from build123d import *

# Parameters (mm, degrees)
BOX008_W               = 22.5
BOX008_H               = 3
BOX008_DEPTH           = 95
BOX009_W               = 6
BOX009_H               = 25
BOX009_DEPTH           = 95
CYLINDER012_R          = 12.5
CYLINDER012_DEPTH      = 13
CYLINDER012_ROLL_ANGLE = 90


with BuildPart() as cube008:
    # Box008 → Box008 (new body)
    with BuildSketch(Plane(origin=(-7.5, 19, 0), x_dir=(1, 0, 0), z_dir=(0, 0, 1))):
        with Locations((11.25, 1.5)):
            Rectangle(BOX008_W, BOX008_H)
    extrude(amount=BOX008_DEPTH)


with BuildPart() as cube009:
    # Box009 → Box009 (new body)
    with BuildSketch(Plane(origin=(0.75, 0, 0), x_dir=(1, 0, 0), z_dir=(0, 0, 1))):
        with Locations((3, 12.5)):
            Rectangle(BOX009_W, BOX009_H)
    extrude(amount=BOX009_DEPTH)


with BuildPart() as obj1:
    # Cylinder012 → Cylinder012 (new body)
    with BuildSketch(Plane.XY):
        Circle(CYLINDER012_R)
    extrude(amount=CYLINDER012_DEPTH)


with BuildPart() as obj1_1:
    # Cylinder012 roll: moved
    add(obj1.part.rotate(Axis((0, 0, 0), (1, 0, 0)), CYLINDER012_ROLL_ANGLE))


with BuildPart() as obj1_2:
    # Cylinder012 placement: moved
    add(obj1_1.part.moved(Location((3.75, 22, 96.2))))

    # Fusion017: union Cube008, Cube009
    add(cube008.part)
    add(cube009.part)


solid = obj1_2.part
Verification items for the finished model (mm, model axes). A direction names the side the tool comes from. Coordinates: 2 decimals unless noted, no trailing zeros. Loops run counter-clockwise (first coordinate to the right, second up) from the corner with the lowest first, then second, coordinate; pieces in that order, holes last. Notation, with made-up numbers: M 43,13 L 90,13 A5 cw 90,22 Z; hole C -30.5,56 d11. An arc over 180 degrees is marked long. One line per item, written item: value.
1. Section check D-D on x = 11.25. Record the cut outline in (y, z), plus the area to 3 significant figures.
Answers follow:
outline: M 9,86.2 L 19,86.2 L 19,0 L 22,0 L 22,106.2 L 9,106.2 Z
area: 519 mm^2
2. Set-up check for faces 1 (the flat face through (-3, 19, 45)), 2 (the flat face through (0.75, 23, 47)), 3 (the flat face through (6.75, 9, 47)): record each of +Z, -Z, +X, -X, +Y, -Y from which the full face is reachable in a straight line by a thin tool's end or side.
Answers follow:
face 1: -Z, -X, -Y
face 2: +Z, -Z, -X, +Y
face 3: -Z, +X, -Y
3. Section check A-A on z = 12. Record the cut outline in (x, y), plus the area to 4 significant figures.
Answers follow:
outline: M -7.5,19 L 0.75,19 L 0.75,0 L 6.75,0 L 6.75,19 L 15,19 L 15,22 L 6.75,22 L 6.75,25 L 0.75,25 L 0.75,22 L -7.5,22 Z
area: 199.5 mm^2
4. Gauge pin test, flat ends, axial feed: P1, Ø0.9, axis at y = 23, z = 61.5, coming from the -X side; P2, Ø1, axis at x = 13.5, y = 20.5, coming from the +Z side; P3, Ø7.5, axis at x = 4, z = 97, coming from the -Y side; P4, Ø1, axis at x = 7.5, y = 12.5, coming from the -Z side. Record the tip position at first contact, or that the pin passes through.
Answers follow:
P1: x = 0.75
P2: z = 104.61
P3: y = 0
P4: z = 84.13
5. Section check B-B on x = 3.75. Record the cut outline in (y, z), plus the area to 3 significant figures.
Answers follow:
outline: M 0,0 L 25,0 L 25,95 L 22,95 L 22,108.7 L 9,108.7 L 9,95 L 0,95 Z
area: 2,550 mm^2
6. Section check C-C on y = 5.5. Record the cut outline in (x, z).
Answers follow:
outline: M 0.75,0 L 6.75,0 L 6.75,95 L 0.75,95 Z
7. Material ranges on line 1 along X through (y, z) = (8, 67.5); line 2 along Z through (x, y) = (5, 4); line 3 along Y through (x, z) = (-3, 76), recorded low to high. Write a range as from..to.
Answers follow:
line 1: 0.75..6.75
line 2: 0..95
line 3: 19..22
